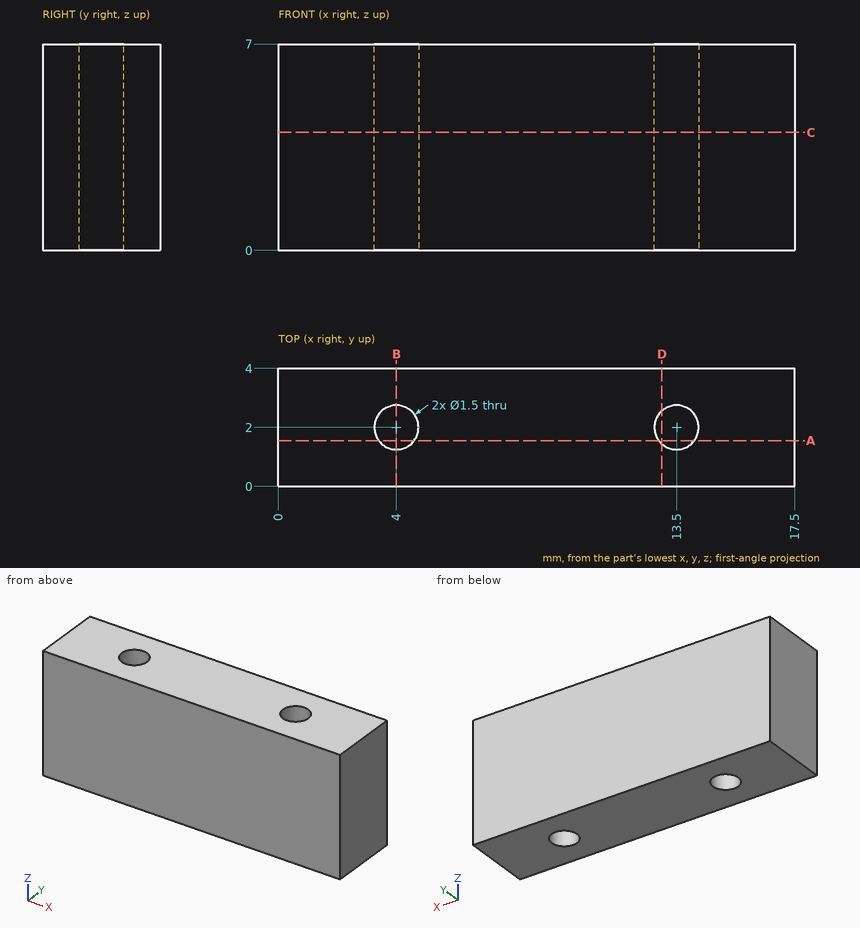
Input: dimensioned drawing with shaded views. Units: mm. Origin: part minimum x, y, z. Round coordinates to 2 decimals unless told otherwise and drop trailing zeros. Write each loop counter-clockwise with the first axis right and the second up, starting at its lowest first coordinate (ties: lowest second). Pieces come first, ordered by that corner, then holes. Notation, with made-up numbers: (81, -39) -> (89, -39) arc R16 ccw to (89, -9) -> close; hole circle Ø11 at (23, 24). An arc over 180 degrees is marked (long way). Use CSV: the item, a comma, the result in double quotes. Start each with the question number.
Q1. Line query: L1, parallel to Y at x = 13.5, z = 4; L2, parallel to X at y = 2.65, z = 3.5; L3, parallel to X at y = 1.6, z = 5. Output: solid intervals per line, ascending.
Q2. Section A-A (y = 1.55). Return loops of the section in (x, z), plus the area to 3 significant figures.
Q3. Section B-B (x = 4). Return loops of the section in (y, z).
Q4. Section C-C (z = 4). Return loops of the section in (x, y), plus the area to 3 significant figures.
Q5. Section D-D (x = 13). Return loops of the section in (y, z), plus the area to 3 significant figures.
Result sheet:
1,L1,"0 to 1.25, 2.75 to 4"
1,L2,"0 to 3.63, 4.37 to 13.13, 13.87 to 17.5"
1,L3,"0 to 3.37, 4.63 to 12.87, 14.13 to 17.5"
2,outline,"(0, 0) -> (3.4, 0) -> (3.4, 7) -> (0, 7) -> close; (4.6, 0) -> (12.9, 0) -> (12.9, 7) -> (4.6, 7) -> close; (14.1, 0) -> (17.5, 0) -> (17.5, 7) -> (14.1, 7) -> close"
2,area,"106 mm²"
3,outline,"(0, 0) -> (1.25, 0) -> (1.25, 7) -> (0, 7) -> close; (2.75, 0) -> (4, 0) -> (4, 7) -> (2.75, 7) -> close"
4,outline,"(0, 0) -> (17.5, 0) -> (17.5, 4) -> (0, 4) -> close; hole circle Ø1.5 at (4, 2); hole circle Ø1.5 at (13.5, 2)"
4,area,"66.5 mm²"
5,outline,"(0, 0) -> (1.44, 0) -> (1.44, 7) -> (0, 7) -> close; (2.56, 0) -> (4, 0) -> (4, 7) -> (2.56, 7) -> close"
5,area,"20.2 mm²"
